The listing builds one solid part. Answer for the finished solid, in the listing's coordinates (mm). A direction names the side the tool comes from. Round coordinates to 2 decimals unless told otherwise and drop trailing zeros. Order: outer loops, then holes, each group sorted by start corner. A loop starts at its lowest first (then second) coordinate and runs counter-clockwise, first axis right, second up. Notation, with made-up numbers: (22, 46.25) - (77, 46.25) arc R10 cw to (77, 61.25) - close; hole circle Ø10 at (52, 71). An arc over 180 degrees is marked (long way). One line per item, written item: value. Start each with the question number.
1. Section C-C, the plane x = 102 is taken. Give the vertices of the cut face in (y, z).
2. Straight lines are drawn through the part: line 1 (X direction, y = 10, z = 40); line 2 (X direction, y = 90, z = 43); line 3 (Y direction, x = 10, z = 43.75). For each, find the intervals that lie inside material, in ascending order.
3. Section D-D, the plane z = 14 is taken. Give the vertices of the cut face in (x, y).
4. A tool of negligible diameter and unlimited length cuts with its end or side. For faces 4 (the flat face through (88.934, 89.938, 23.035)), 5 (the cylindrical face through (90, 13, 10)), 6 (the flat face through (88.95, 14.4, 7.45)), from which of +Z, -Z, +X, -X, +Y, -Y can it reach the whole face along a straight path? Write none if from no direction.
5. For a pull along X with two mould halves and no side action, classify faces 1 (the flat face through (157.36, 50.59, 22.84)), 2 (the flat face through (83, 94, 47)), 3 (the flat face through (88.95, 88.503, 21.054)) as released by +X, released by -X, zero draft, split by the parting line, or undercut.
6. Flat-ended cylindrical pins translate along their axes: P1, Ø0.7, axis at y = 58.5, z = 46.5, coming from the -X side; P2, Ø4, axis at x = 42.5, y = 35, coming from the -Z side; P3, Ø1, axis at y = 58.5, z = 46.5, coming from the +X side; P4, Ø0.9, axis at x = 159, z = 46.5, coming from the -Y side. Find the tip coordinate at first contact, or state that the pin passes through.
7. Section B-B, the plane y = 71.5 is taken. Give the vertices of the cut face in (x, z), then the cut area to 3 significant figures.
8. Section A-A, the plane x = 170 is taken. Count the separate pieces of the cut face and the enclosed holes in it, then the cut area to 3 significant figures.
from build123d import *

# Parameters (mm, degrees)
BOX020_W               = 50
BOX020_H               = 20
BOX020_DEPTH           = 25
CYLINDER004_R          = 25
CYLINDER004_DEPTH      = 20
CYLINDER004_ROLL_ANGLE = 90
BOX019_W               = 120
BOX019_H               = 10
BOX019_DEPTH           = 10
CYLINDER003_R          = 2.25
CYLINDER003_DEPTH      = 60
CYLINDER002_R          = 2.25
CYLINDER002_DEPTH      = 60
CYLINDER001_R          = 2.25
CYLINDER001_DEPTH      = 60
CYLINDER_R             = 2.25
CYLINDER_DEPTH         = 60
BOX018_W               = 180
BOX018_H               = 50
BOX018_DEPTH           = 60
BOX018_ROLL_ANGLE      = -12.3
BOX017_W               = 180
BOX017_H               = 50
BOX017_DEPTH           = 60
BOX017_ROLL_ANGLE      = 12.3
BOX016_W               = 70
BOX016_H               = 100
BOX016_DEPTH           = 50
BOX016_PITCH_ANGLE     = 52.5
BOX015_W               = 70
BOX015_H               = 100
BOX015_DEPTH           = 50
BOX015_PITCH_ANGLE     = -52.5
BOX007_W               = 100
BOX007_H               = 70
BOX007_DEPTH           = 1
BOX014_W               = 170
BOX014_H               = 2
BOX014_DEPTH           = 7
BOX013_W               = 170
BOX013_H               = 2
BOX013_DEPTH           = 7
BOX012_W               = 2
BOX012_H               = 80
BOX012_DEPTH           = 2.5
BOX011_W               = 2
BOX011_H               = 80
BOX011_DEPTH           = 2.5
BOX010_W               = 10
BOX010_H               = 10
BOX010_DEPTH           = 13
BOX009_W               = 10
BOX009_H               = 10
BOX009_DEPTH           = 13
BOX008_W               = 10
BOX008_H               = 10
BOX008_DEPTH           = 13
BOX_W                  = 10
BOX_H                  = 10
BOX_DEPTH              = 13
BOX005_W               = 180
BOX005_H               = 1
BOX005_DEPTH           = 47
BOX005_ROLL_ANGLE      = -12.3
BOX004_W               = 180
BOX004_H               = 1
BOX004_DEPTH           = 47
BOX004_ROLL_ANGLE      = 12.3
BOX003_W               = 58
BOX003_H               = 100
BOX003_DEPTH           = 1
BOX003_PITCH_ANGLE     = -52.5
BOX002_W               = 58
BOX002_H               = 100
BOX002_DEPTH           = 1
BOX002_PITCH_ANGLE     = 52.5


with BuildPart() as cube020:
    # Box020 → Box020 (new body)
    with BuildSketch(Plane(origin=(65, 0, 35), x_dir=(1, 0, 0), z_dir=(0, 0, 1))):
        with Locations((25, 10)):
            Rectangle(BOX020_W, BOX020_H)
    extrude(amount=BOX020_DEPTH)


with BuildPart() as cylinder:
    # Cylinder004 → Cylinder004 (new body)
    with BuildSketch(Plane.XY):
        Circle(CYLINDER004_R)
    extrude(amount=CYLINDER004_DEPTH)


with BuildPart() as cylinder_1:
    # Cylinder004 roll: moved
    add(cylinder.part.rotate(Axis((0, 0, 0), (1, 0, 0)), CYLINDER004_ROLL_ANGLE))


with BuildPart() as cylinder_2:
    # Cylinder004 placement: moved
    add(cylinder_1.part.moved(Location((90, 20, 35))))


with BuildPart() as cube019:
    # Box019 → Box019 (new body)
    with BuildSketch(Plane(origin=(30, 0, 43), x_dir=(1, 0, 0), z_dir=(0, 0, 1))):
        with Locations((60, 5)):
            Rectangle(BOX019_W, BOX019_H)
    extrude(amount=BOX019_DEPTH)


with BuildPart() as cylinder003:
    # Cylinder003 → Cylinder003 (new body)
    with BuildSketch(Plane(origin=(170, 90, 0), x_dir=(1, 0, 0), z_dir=(0, 0, 1))):
        Circle(CYLINDER003_R)
    extrude(amount=CYLINDER003_DEPTH)


with BuildPart() as cylinder002:
    # Cylinder002 → Cylinder002 (new body)
    with BuildSketch(Plane(origin=(10, 90, 0), x_dir=(1, 0, 0), z_dir=(0, 0, 1))):
        Circle(CYLINDER002_R)
    extrude(amount=CYLINDER002_DEPTH)


with BuildPart() as cylinder001:
    # Cylinder001 → Cylinder001 (new body)
    with BuildSketch(Plane(origin=(170, 10, 0), x_dir=(1, 0, 0), z_dir=(0, 0, 1))):
        Circle(CYLINDER001_R)
    extrude(amount=CYLINDER001_DEPTH)


with BuildPart() as cylinder000:
    # Cylinder → Cylinder (new body)
    with BuildSketch(Plane(origin=(10, 10, 0), x_dir=(1, 0, 0), z_dir=(0, 0, 1))):
        Circle(CYLINDER_R)
    extrude(amount=CYLINDER_DEPTH)


with BuildPart() as cube018:
    # Box018 → Box018 (new body)
    with BuildSketch(Plane.XY):
        with Locations((90, 25)):
            Rectangle(BOX018_W, BOX018_H)
    extrude(amount=BOX018_DEPTH)


with BuildPart() as cube018_1:
    # Box018 roll: moved
    add(cube018.part.rotate(Axis((0, 0, 0), (1, 0, 0)), BOX018_ROLL_ANGLE))


with BuildPart() as cube018_2:
    # Box018 placement: moved
    add(cube018_1.part.moved(Location((1, 84, -4.2))))


with BuildPart() as cube017:
    # Box017 → Box017 (new body)
    with BuildSketch(Plane.XY):
        with Locations((90, 25)):
            Rectangle(BOX017_W, BOX017_H)
    extrude(amount=BOX017_DEPTH)


with BuildPart() as cube017_1:
    # Box017 roll: moved
    add(cube017.part.rotate(Axis((0, 0, 0), (1, 0, 0)), BOX017_ROLL_ANGLE))


with BuildPart() as cube017_2:
    # Box017 placement: moved
    add(cube017_1.part.moved(Location((1, -32.9, -15))))


with BuildPart() as cube016:
    # Box016 → Box016 (new body)
    with BuildSketch(Plane.XY):
        with Locations((35, 50)):
            Rectangle(BOX016_W, BOX016_H)
    extrude(amount=BOX016_DEPTH)


with BuildPart() as cube016_1:
    # Box016 pitch: moved
    add(cube016.part.rotate(Axis((0, 0, 0), (0, 1, 0)), BOX016_PITCH_ANGLE))


with BuildPart() as cube016_2:
    # Box016 placement: moved
    add(cube016_1.part.moved(Location((-39.5, 0, 22))))


with BuildPart() as cube015:
    # Box015 → Box015 (new body)
    with BuildSketch(Plane.XY):
        with Locations((35, 50)):
            Rectangle(BOX015_W, BOX015_H)
    extrude(amount=BOX015_DEPTH)


with BuildPart() as cube015_1:
    # Box015 pitch: moved
    add(cube015.part.rotate(Axis((0, 0, 0), (0, 1, 0)), BOX015_PITCH_ANGLE))


with BuildPart() as cube015_2:
    # Box015 placement: moved
    add(cube015_1.part.moved(Location((176, 0, -35))))


with BuildPart() as cube007:
    # Box007 → Box007 (new body)
    with BuildSketch(Plane(origin=(40, 15, 0), x_dir=(1, 0, 0), z_dir=(0, 0, 1))):
        with Locations((50, 35)):
            Rectangle(BOX007_W, BOX007_H)
    extrude(amount=BOX007_DEPTH)


with BuildPart() as cube014:
    # Box014 → Box014 (new body)
    with BuildSketch(Plane(origin=(5, 93, 40), x_dir=(1, 0, 0), z_dir=(0, 0, 1))):
        with Locations((85, 1)):
            Rectangle(BOX014_W, BOX014_H)
    extrude(amount=BOX014_DEPTH)


with BuildPart() as cube013:
    # Box013 → Box013 (new body)
    with BuildSketch(Plane(origin=(5, 5, 40), x_dir=(1, 0, 0), z_dir=(0, 0, 1))):
        with Locations((85, 1)):
            Rectangle(BOX013_W, BOX013_H)
    extrude(amount=BOX013_DEPTH)


with BuildPart() as cube012:
    # Box012 → Box012 (new body)
    with BuildSketch(Plane(origin=(173, 5, 44.5), x_dir=(1, 0, 0), z_dir=(0, 0, 1))):
        with Locations((1, 40)):
            Rectangle(BOX012_W, BOX012_H)
    extrude(amount=BOX012_DEPTH)


with BuildPart() as cube011:
    # Box011 → Box011 (new body)
    with BuildSketch(Plane(origin=(5, 5, 44.5), x_dir=(1, 0, 0), z_dir=(0, 0, 1))):
        with Locations((1, 40)):
            Rectangle(BOX011_W, BOX011_H)
    extrude(amount=BOX011_DEPTH)


with BuildPart() as cube010:
    # Box010 → Box010 (new body)
    with BuildSketch(Plane(origin=(5, 85, 34), x_dir=(1, 0, 0), z_dir=(0, 0, 1))):
        with Locations((5, 5)):
            Rectangle(BOX010_W, BOX010_H)
    extrude(amount=BOX010_DEPTH)


with BuildPart() as cube009:
    # Box009 → Box009 (new body)
    with BuildSketch(Plane(origin=(165, 85, 34), x_dir=(1, 0, 0), z_dir=(0, 0, 1))):
        with Locations((5, 5)):
            Rectangle(BOX009_W, BOX009_H)
    extrude(amount=BOX009_DEPTH)


with BuildPart() as cube008:
    # Box008 → Box008 (new body)
    with BuildSketch(Plane(origin=(165, 5, 34), x_dir=(1, 0, 0), z_dir=(0, 0, 1))):
        with Locations((5, 5)):
            Rectangle(BOX008_W, BOX008_H)
    extrude(amount=BOX008_DEPTH)


with BuildPart() as cube:
    # Box → Box (new body)
    with BuildSketch(Plane(origin=(5, 5, 34), x_dir=(1, 0, 0), z_dir=(0, 0, 1))):
        with Locations((5, 5)):
            Rectangle(BOX_W, BOX_H)
    extrude(amount=BOX_DEPTH)


with BuildPart() as cube005:
    # Box005 → Box005 (new body)
    with BuildSketch(Plane.XY):
        with Locations((90, 0.5)):
            Rectangle(BOX005_W, BOX005_H)
    extrude(amount=BOX005_DEPTH)


with BuildPart() as cube005_1:
    # Box005 roll: moved
    add(cube005.part.rotate(Axis((0, 0, 0), (1, 0, 0)), BOX005_ROLL_ANGLE))


with BuildPart() as cube005_2:
    # Box005 placement: moved
    add(cube005_1.part.moved(Location((1, 84, 0.4))))


with BuildPart() as fusion001:
    # Box004 → Box004 (new body)
    with BuildSketch(Plane.XY):
        with Locations((90, 0.5)):
            Rectangle(BOX004_W, BOX004_H)
    extrude(amount=BOX004_DEPTH)


with BuildPart() as fusion001_1:
    # Box004 roll: moved
    add(fusion001.part.rotate(Axis((0, 0, 0), (1, 0, 0)), BOX004_ROLL_ANGLE))


with BuildPart() as fusion001_2:
    # Box004 placement: moved
    add(fusion001_1.part.moved(Location((1, 15, 0))))

    # Fusion001: union Cube005
    add(cube005_2.part)


with BuildPart() as cube003:
    # Box003 → Box003 (new body)
    with BuildSketch(Plane.XY):
        with Locations((29, 50)):
            Rectangle(BOX003_W, BOX003_H)
    extrude(amount=BOX003_DEPTH)


with BuildPart() as cube003_1:
    # Box003 pitch: moved
    add(cube003.part.rotate(Axis((0, 0, 0), (0, 1, 0)), BOX003_PITCH_ANGLE))


with BuildPart() as cube003_2:
    # Box003 placement: moved
    add(cube003_1.part.moved(Location((140, 0, 0.1))))


with BuildPart() as cut010:
    # Box002 → Box002 (new body)
    with BuildSketch(Plane.XY):
        with Locations((29, 50)):
            Rectangle(BOX002_W, BOX002_H)
    extrude(amount=BOX002_DEPTH)


with BuildPart() as cut010_1:
    # Box002 pitch: moved
    add(cut010.part.rotate(Axis((0, 0, 0), (0, 1, 0)), BOX002_PITCH_ANGLE))


with BuildPart() as cut010_2:
    # Box002 placement: moved
    add(cut010_1.part.moved(Location((5, 0, 46))))

    # Fusion: union Cube003
    add(cube003_2.part)

    # Fusion002: union Fusion001
    add(fusion001_2.part)

    # Fusion003: union Cube
    add(cube.part)

    # Fusion004: union Cube008
    add(cube008.part)

    # Fusion005: union Cube009
    add(cube009.part)

    # Fusion006: union Cube010
    add(cube010.part)

    # Fusion007: union Cube011
    add(cube011.part)

    # Fusion008: union Cube012
    add(cube012.part)

    # Fusion009: union Cube013
    add(cube013.part)

    # Fusion010: union Cube014
    add(cube014.part)

    # Fusion011: union Cube007
    add(cube007.part)

    # Cut: cut Cube015
    add(cube015_2.part, mode=Mode.SUBTRACT)

    # Cut001: cut Cube016
    add(cube016_2.part, mode=Mode.SUBTRACT)

    # Cut002: cut Cube017
    add(cube017_2.part, mode=Mode.SUBTRACT)

    # Cut003: cut Cube018
    add(cube018_2.part, mode=Mode.SUBTRACT)

    # Cut004: cut Cylinder000
    add(cylinder000.part, mode=Mode.SUBTRACT)

    # Cut005: cut Cylinder001
    add(cylinder001.part, mode=Mode.SUBTRACT)

    # Cut006: cut Cylinder002
    add(cylinder002.part, mode=Mode.SUBTRACT)

    # Cut007: cut Cylinder003
    add(cylinder003.part, mode=Mode.SUBTRACT)

    # Cut008: cut Cube019
    add(cube019.part, mode=Mode.SUBTRACT)

    # Cut009: cut Cylinder
    add(cylinder_2.part, mode=Mode.SUBTRACT)

    # Cut010: cut Cube020
    add(cube020.part, mode=Mode.SUBTRACT)


solid = cut010_2.part
Answer list:
1. outline: (12.15, 13.07) - (15, 0) - (84.92, 0) - (95, 46.25) - (95, 47) - (93, 47) - (93, 41.68) - (84.13, 1) - (15.81, 1) - (13.17, 13.07) - close
2. line 1: x = 12.25 to 15, 165 to 167.75
2. line 2: x = 7.41 to 7.75, 12.25 to 15, 165 to 167.75, 172.25 to 172.83
2. line 3: y = 5.47 to 7.75, 12.25 to 15, 85 to 87.75, 92.25 to 94.45
3. outline: (29.66, 11.95) - (76.44, 11.95) - (76.44, 12.97) - (30.81, 12.97) - (30.81, 86.97) - (149.41, 86.97) - (149.41, 12.97) - (103.56, 12.97) - (103.56, 11.95) - (150.58, 11.95) - (150.58, 87.97) - (29.66, 87.97) - close
4. face 4: -Z, +X, -X, +Y
4. face 5: +Z, -Y
4. face 6: +Z
5. face 1: released by +X
5. face 2: zero draft
5. face 3: undercut
6. P1: stops at x = 5
6. P2: stops at z = 0
6. P3: stops at x = 175.25
6. P4: stops at y = 5
7. outline: (5, 46.14) - (40.4, 0) - (139.83, 0) - (175.25, 46.16) - (175, 46.35) - (175, 47) - (173, 47) - (173, 44.75) - (139.43, 1) - (40.79, 1) - (7, 45.04) - (7, 47) - (5, 47) - close
7. area: 210 mm²
8. separate pieces: 3
8. enclosed holes: 0
8. area: 181 mm²
